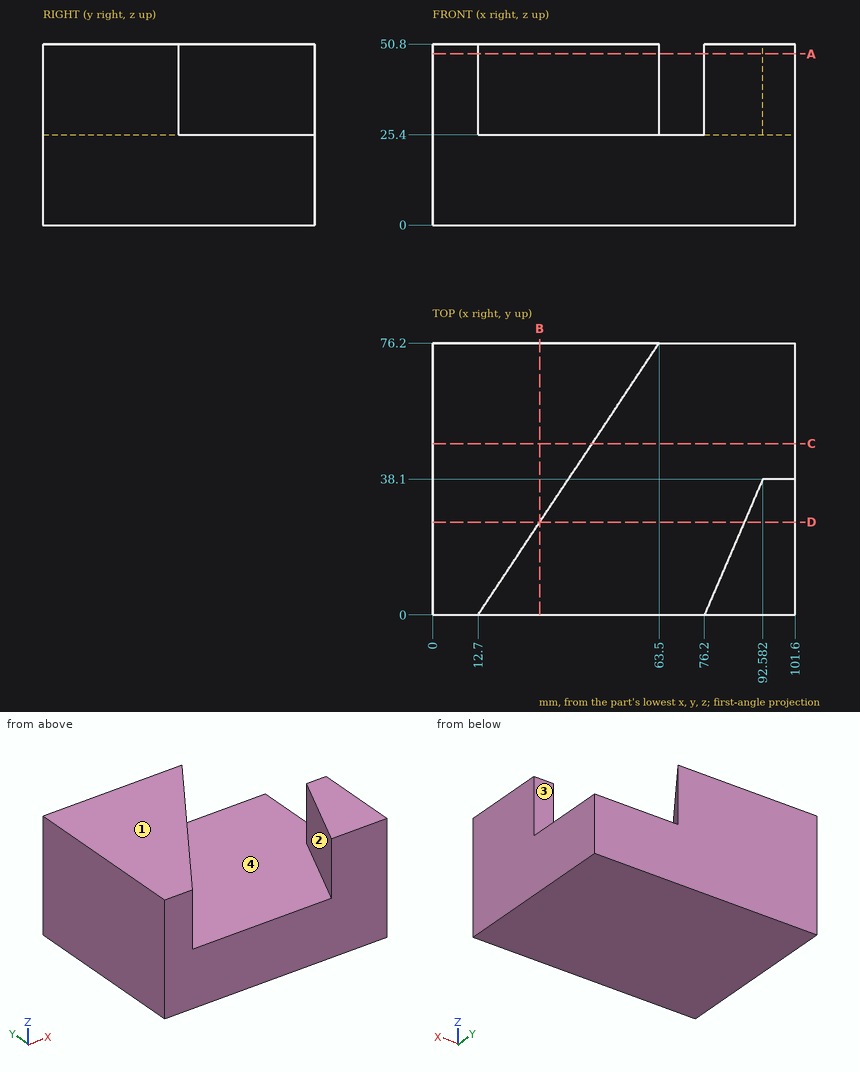
Study the drawing (mm; zero at the part's minimum x, y, z) and answer. A direction names the side the tool comes from. Give positions to 0.01 mm unless a question says otherwise; leave off trailing zeros. Order: outer loops, then holes, each group sorted by start corner. A loop starts at its lowest first (then second) coordinate and runs counter-clockwise, first axis right, second up.
1. Section B-B, the plane x = 30 is taken. Determine the outline of the cut face in (y, z), and give its area (3 significant figures).
Result sheet:
outline: (0, 0) - (76.2, 0) - (76.2, 50.8) - (25.95, 50.8) - (25.95, 25.4) - (0, 25.4) - close
area: 3,210 mm2
2. Each of these flat-tipped pins is pushed along its axis until it touches: P1, Ø1.5, axis at x = 31, y = 18, coming from the +Z side; P2, Ø2.5, axis at x = 98, z = 32, coming from the +Y side; P3, Ø1, axis at y = 53, z = 44, coming from the +X side. Where does it stop, or does it pass through?
Result sheet:
P1: stops at z = 25.4
P2: stops at y = 38.1
P3: stops at x = 48.37
3. Section C-C, the plane y = 48 is taken. Determine the outline of the cut face in (x, z).
Result sheet:
outline: (0, 0) - (101.6, 0) - (101.6, 25.4) - (44.7, 25.4) - (44.7, 50.8) - (0, 50.8) - close
4. Straight lines are drawn through the part: L1, parallel to Z at x = 81, y = 33.5; L2, parallel to X at y = 5, z = 47; L3, parallel to X at y = 10, z = 43. For each, find the intervals that lie inside material, in ascending order.
Result sheet:
L1: z = 0 to 25.4
L2: x = 0 to 16.03, 78.35 to 101.6
L3: x = 0 to 19.37, 80.5 to 101.6
5. For the marked faces 1, 2, 3 and 4, determine the directions among +Z, -Z, +X, -X, +Y, -Y from which every point of the face is accessible in a straight line to the end or side of a thin tool.
Result sheet:
face 1: +Z, +X, -X, +Y, -Y
face 2: +Z, +Y
face 3: +Z, +X, +Y
face 4: +Z
6. Section A-A, the plane z = 48 is taken. Determine the outline of the cut face in (x, y), and give its area (3 significant figures).
Result sheet:
outline: (0, 0) - (12.7, 0) - (63.5, 76.2) - (0, 76.2) - close; (76.2, 0) - (101.6, 0) - (101.6, 38.1) - (92.58, 38.1) - close
area: 3,560 mm2
7. Section D-D, the plane y = 26 is taken. Determine the outline of the cut face in (x, z), and give its area (3 significant figures).
Result sheet:
outline: (0, 0) - (101.6, 0) - (101.6, 50.8) - (87.38, 50.8) - (87.38, 25.4) - (30.03, 25.4) - (30.03, 50.8) - (0, 50.8) - close
area: 3,700 mm2
